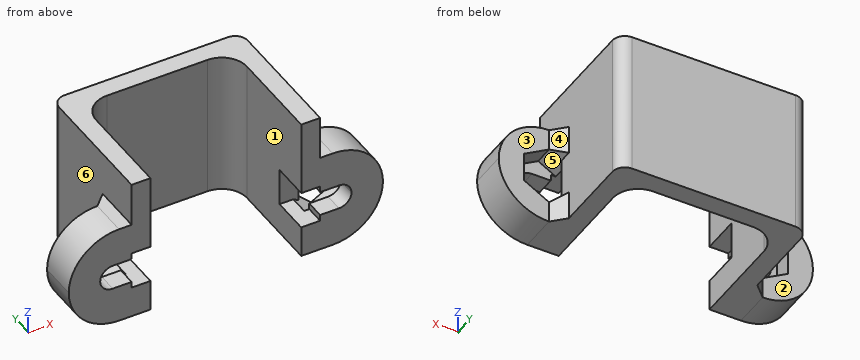
from build123d import *

# Parameters (mm, degrees)
SKETCH_1_W          = 15
SKETCH_1_H          = 11
EXTRUDE_1_DEPTH     = 11.5
SKETCH_2_W          = 5
SKETCH_2_H          = 8
EXTRUDE_2_DEPTH     = 3
SKETCH_3_W          = 12
SKETCH_3_H          = 9.5
CUT_EXTRUDE_1_DEPTH = 21.236106345
CUT_EXTRUDE_2_DEPTH = 1.5
SKETCH_5_W          = 1.5
SKETCH_5_H          = 3
CUT_EXTRUDE_3_DEPTH = 3
SKETCH_6_W          = 2.5
SKETCH_6_H          = 2
CUT_EXTRUDE_4_DEPTH = 1.5
FILLET_1_R          = 2
FILLET_2_R          = 4
FILLET_3_R          = 1
CHAMFER_1_SIZE      = 1
FILLET_4_R          = 1


with BuildPart() as part:
    # 草图1 → 凸台-拉伸1 (new body)
    with BuildSketch(Plane.XY):
        with Locations((0, 5.5)):
            Rectangle(SKETCH_1_W, SKETCH_1_H)
    extrude(amount=EXTRUDE_1_DEPTH)

    # 草图2 → 凸台-拉伸2 (add)
    with BuildSketch(Plane.XZ):
        with Locations((-10, 4)):
            Rectangle(SKETCH_2_W, SKETCH_2_H)
        with Locations((10, 4)):
            Rectangle(SKETCH_2_W, SKETCH_2_H)
    extrude(amount=-EXTRUDE_2_DEPTH)

    # 草图3 → 切除-拉伸1 (cut, through all)
    with BuildSketch(Plane(origin=(0, 0, 0), x_dir=(-1, 0, 0), z_dir=(0, 0, -1))):
        with Locations((0, 4.75)):
            Rectangle(SKETCH_3_W, SKETCH_3_H)
    extrude(amount=-CUT_EXTRUDE_1_DEPTH, mode=Mode.SUBTRACT)

    # 草图4 → 切除-拉伸2 (cut)
    with BuildSketch(Plane(origin=(0, 3, 0), x_dir=(1, 0, 0), z_dir=(0, 1, 0))):
        Polygon((8.5, -1.690598923), (6.5, -2.845299462), (6.5, -5.154700538), (8.5, -6.309401077), (10.5, -5.154700538), (10.5, -2.845299462), align=None)
        Polygon((-10.5, -2.845299462), (-8.5, -1.690598923), (-6.5, -2.845299462), (-6.5, -5.154700538), (-8.5, -6.309401077), (-10.5, -5.154700538), align=None)
    extrude(amount=-CUT_EXTRUDE_2_DEPTH, mode=Mode.SUBTRACT)

    # 草图5 → 切除-拉伸3 (cut)
    with BuildSketch(Plane.XZ):
        with Locations((6.75, 4)):
            Rectangle(SKETCH_5_W, SKETCH_5_H)
        with Locations((-6.75, 4)):
            Rectangle(SKETCH_5_W, SKETCH_5_H)
    extrude(amount=-CUT_EXTRUDE_3_DEPTH, mode=Mode.SUBTRACT)

    # 草图6 → 切除-拉伸4 (cut)
    with BuildSketch(Plane.XZ):
        with Locations((8.75, 4)):
            Rectangle(SKETCH_6_W, SKETCH_6_H)
        with Locations((-8.75, 4)):
            Rectangle(SKETCH_6_W, SKETCH_6_H)
    extrude(amount=-CUT_EXTRUDE_4_DEPTH, mode=Mode.SUBTRACT)

    # 圆角1
    fillet_1_edges = [part.edges().sort_by_distance(p)[0] for p in [
        (6, 9.5, 5.75),
        (-6, 9.5, 5.75),
    ]]
    fillet(fillet_1_edges, radius=FILLET_1_R)

    # 圆角2
    fillet_2_edges = [part.edges().sort_by_distance(p)[0] for p in [
        (12.5, 1.5, 0),
        (12.5, 1.5, 8),
        (-12.5, 1.5, 0),
        (-12.5, 1.5, 8),
    ]]
    fillet(fillet_2_edges, radius=FILLET_2_R - 0.0001)  # a hair under: the kernel refuses the full size

    # 圆角3
    fillet_3_edges = [part.edges().sort_by_distance(p)[0] for p in [
        (10, 0.75, 5),
        (10, 0.75, 3),
        (-10, 0.75, 3),
        (-10, 0.75, 5),
    ]]
    fillet(fillet_3_edges, radius=FILLET_3_R - 0.0001)  # a hair under: the kernel refuses the full size

    # 倒角1
    chamfer_1_edges = [part.edges().sort_by_distance(p)[0] for p in [
        (7.5, 3, 6.866025404),
        (7.5, 3, 1.133974596),
        (-7.5, 3, 6.866025404),
        (-7.5, 3, 1.133974596),
    ]]
    chamfer(chamfer_1_edges, length=CHAMFER_1_SIZE)

    # 圆角4
    fillet_4_edges = [part.edges().sort_by_distance(p)[0] for p in [
        (-7.5, 11, 5.75),
        (7.5, 11, 5.75),
    ]]
    fillet(fillet_4_edges, radius=FILLET_4_R)


solid = part.part
Geometry check sheet. Reference: the model listing, model coordinates, mm. Face numbers are marked on the shaded views. A direction names the side the tool comes from. Give positions to 0.01 mm unless a question says otherwise; leave off trailing zeros. Loops run counter-clockwise (first coordinate to the right, second up) from the corner with the lowest first, then second, coordinate; pieces in that order, holes last. Notation, with made-up numbers: (15.5, -6.75) -> (40.5, -6.75) arc R20 cw to (40.5, 17.25) -> close; hole circle Ø5 at (1.25, 55). An arc over 180 degrees is marked (long way). Answer in a Markdown table with one row per item. Add a question column.
1) Cross-section at A-A on y = 5.5. Record the boundary of the cut face in (x, z).
2) Gauge pin test, flat ends, axial feed: P1, Ø1.5, axis at x = 8, z = 4.5, coming from the +Y side; P2, Ø5, axis at y = 1, z = 8, coming from the +X side; P3, Ø0.8, axis at x = -8, y = 1, coming from the +Z side. Record the tip position at first contact, or that the pin passes through.
3) Cross-section at C-C on x = 8.25. Record the boundary of the cut face in (y, z), and give its area (3 significant figures).
4) Cross-section at B-B on z = 10.75. Record the boundary of the cut face in (x, y).
5) Material ranges on probe 1 along X at (y, z) = (3.5, 8.75); probe 2 along X at (y, z) = (2, 6.25); probe 3 along Y at (x, z) = (-2.5, 3.5), recorded low to high. Write a range as from..to.
6) Cross-section at D-D on x = -2. Record the boundary of the cut face in (y, z), and give its area (4 significant figures).
7) Draft check along X on the marked faces 4, 5 and 6. Enter one of: pulls with the +X half, pulls with the -X half, needs draft (parallel to the pull), parting line crosses it, or undercut.
8) Set-up check for the marked faces 1, 2 and 3: record each of +Z, -Z, +X, -X, +Y, -Y from which the full face is reachable in a straight line by a thin tool's end or side.
Outcome:
| question | item | result |
|---|---|---|
| 1 | outline | (-7.5, 0) -> (-6, 0) -> (-6, 11.5) -> (-7.5, 11.5) -> close; (6, 0) -> (7.5, 0) -> (7.5, 11.5) -> (6, 11.5) -> close |
| 2 | P1 | stops at y = 10.66 |
| 2 | P2 | stops at x = 12.21 |
| 2 | P3 | stops at z = 8 |
| 3 | outline | (0, 0) -> (3.25, 0) -> (3.25, 1.83) -> (1.5, 1.83) -> (1.5, 3) -> (0, 3) -> close; (0, 5) -> (1.5, 5) -> (1.5, 6.17) -> (3.25, 6.17) -> (3.25, 8) -> (0, 8) -> close |
| 3 | area | 15.4 mm^2 |
| 4 | outline | (-7.5, 0) -> (-6, 0) -> (-6, 7.5) arc R2 cw to (-4, 9.5) -> (4, 9.5) arc R2 cw to (6, 7.5) -> (6, 0) -> (7.5, 0) -> (7.5, 10) arc R1 ccw to (6.5, 11) -> (-6.5, 11) arc R1 ccw to (-7.5, 10) -> close |
| 5 | probe 1 | x = -7.5..-6, 6..7.5 |
| 5 | probe 2 | x = -11.81..-8.6, -8.4..-6, 6..8.4, 8.6..11.81 |
| 5 | probe 3 | y = 9.5..11 |
| 6 | outline | (9.5, 0) -> (11, 0) -> (11, 11.5) -> (9.5, 11.5) -> close |
| 6 | area | 17.25 mm^2 |
| 7 | face 4 | pulls with the +X half |
| 7 | face 5 | undercut |
| 7 | face 6 | pulls with the -X half |
| 8 | face 1 | +Z, -Z, -Y |
| 8 | face 2 | +Z, -Z, -X, +Y |
| 8 | face 3 | +Z, -Z, +X, +Y |
